from build123d import *

# Parameters (mm, degrees)
SKETCH1_W           = 6
SKETCH1_H           = 6
BOSS_EXTRUDE1_DEPTH = 5.1
SKETCH2_W           = 3
SKETCH2_H           = 3.5
BOSS_EXTRUDE2_DEPTH = 2.4
SKETCH3_R           = 0.35
BOSS_EXTRUDE3_DEPTH = 2


with BuildPart() as part:
    # Sketch1 → Boss-Extrude1 (new body)
    with BuildSketch(Plane(origin=(0, 0, 0), x_dir=(1, 0, 0), z_dir=(0, 1, 0))):
        Rectangle(SKETCH1_W, SKETCH1_H)
    extrude(amount=BOSS_EXTRUDE1_DEPTH)

    # Sketch2 → Boss-Extrude2 (add)
    with BuildSketch(Plane(origin=(0, 5.1, 0), x_dir=(1, 0, 0), z_dir=(0, 1, 0))):
        Rectangle(SKETCH2_W, SKETCH2_H)
    extrude(amount=BOSS_EXTRUDE2_DEPTH)

    # Sketch3 → Boss-Extrude3 (add)
    with BuildSketch(Plane.XZ):
        with Locations(Location((-2.5, 0, 0), (0, 0, 270))):
            Circle(SKETCH3_R)
        with Locations(Location((-2.5, -2, 0), (0, 0, 270))):
            Circle(SKETCH3_R)
        with Locations(Location((-2.5, 2, 0), (0, 0, 270))):
            Circle(SKETCH3_R)
        with Locations(Location((2.5, -2, 0), (0, 0, 90))):
            Circle(SKETCH3_R)
        with Locations(Location((2.5, 0, 0), (0, 0, 90))):
            Circle(SKETCH3_R)
        with Locations(Location((2.5, 2, 0), (0, 0, 90))):
            Circle(SKETCH3_R)
    extrude(amount=BOSS_EXTRUDE3_DEPTH)


solid = part.part
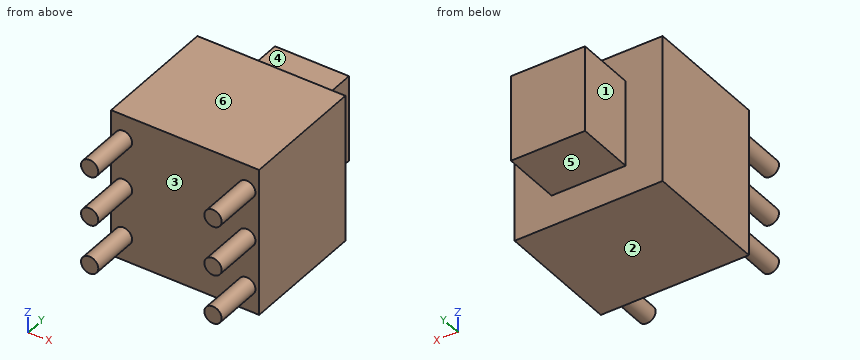
For this review, take the finished solid that the model builds, in its own axes (mm). Face numbers are marked on the shaded views. A direction names the side the tool comes from. Give positions to 0.01 mm unless a question says otherwise; leave off trailing zeros. Order: outer loops, then holes, each group sorted by start corner. A loop starts at its lowest first (then second) coordinate and runs counter-clockwise, first axis right, second up. Notation, with made-up numbers: M 32.5,22.25 L 81.5,22.25 A14 ccw 81.5,36.25 Z; hole C -1,33 d11. An arc over 180 degrees is marked long. Answer in a Markdown table with one row per item. Add a question column.
(1) Mouldability with a two-part tool opening along X and no side actions: class the marked faces 1, 2 and 3 as +X half, -X half, draft (parallel to the pull), parting line (faces both ways), or undercut.
(2) For pin 1 (1.2 mm diameter, centred on y = 6.5, z = 0.5, fed in from -X); pin 2 (1.9 mm diameter, centred on x = 0, y = 6.5, fed in from -Z); pin 3 (1.5 mm diameter, centred on x = -1, z = 1, fed in from -Y), all flat-tipped, find the tip position at first contact; note any pin that passes through.
(3) Consider section C-C on y = -0.25. State the section outline as (x, z) points.
(4) Consider section A-A on x = -0.8. State the section outline as (y, z) points, and give its area (3 significant figures).
(5) Wall thickness on probe 1 along Y at (x, z) = (-0.5, 2.55); probe 2 along Y at (x, z) = (2.65, -1.8); probe 3 along X at (y, z) = (6.25, -0.65): over which ranges is each line inside the solid? List them lowest first. Write a range as [from, to].
(6) For the marked faces 4, 5 and 6, list the 3-axis set-ups (+Z, -Z, +X, -X, +Y, -Y) from which the entire face can be reached by the end or side of a thin tool; tool diameter is ignored.
(7) Consider section B-B on z = 0.55. State the section outline as (x, y) points, and give its area (3 significant figures).
(8) Consider section D-D on y = 5.25. State the section outline as (x, z) points, and give its area (3 significant figures).
Evaluation:
| question | item | result |
|---|---|---|
| 1 | face 1 | -X half |
| 1 | face 2 | draft |
| 1 | face 3 | undercut |
| 2 | pin 1 | stops at x = -1.5 |
| 2 | pin 2 | stops at z = -1.75 |
| 2 | pin 3 | stops at y = 0 |
| 3 | outline | C -2.5,-2 d0.7; C -2.5,0 d0.7; C -2.5,2 d0.7; C 2.5,-2 d0.7; C 2.5,0 d0.7; C 2.5,2 d0.7 |
| 4 | outline | M 0,-3 L 5.1,-3 L 5.1,-1.75 L 7.5,-1.75 L 7.5,1.75 L 5.1,1.75 L 5.1,3 L 0,3 Z |
| 4 | area | 39.0 mm^2 |
| 5 | probe 1 | y = [0, 5.1] |
| 5 | probe 2 | y = [-2, 5.1] |
| 5 | probe 3 | x = [-1.5, 1.5] |
| 6 | face 4 | +Z, +X, -X, +Y |
| 6 | face 5 | -Z, +X, -X, +Y |
| 6 | face 6 | +Z, +X, -X, +Y, -Y |
| 7 | outline | M -3,0 L 3,0 L 3,5.1 L 1.5,5.1 L 1.5,7.5 L -1.5,7.5 L -1.5,5.1 L -3,5.1 Z |
| 7 | area | 37.8 mm^2 |
| 8 | outline | M -1.5,-1.75 L 1.5,-1.75 L 1.5,1.75 L -1.5,1.75 Z |
| 8 | area | 10.5 mm^2 |
